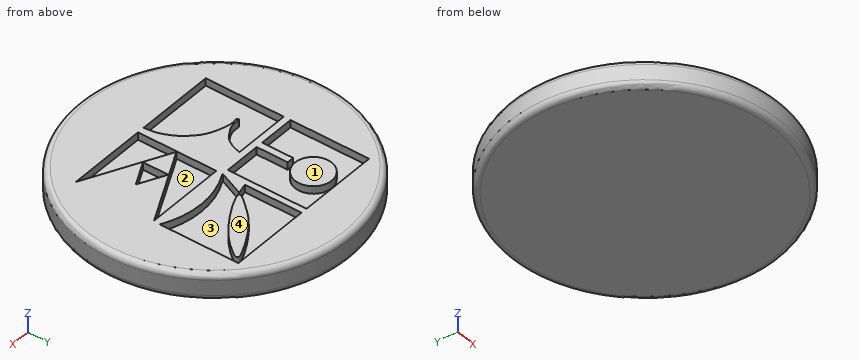
from build123d import *

# Parameters (mm, degrees)
F1_R      = 12.125
F1_W      = 7.0986367516
F1_H      = 7.0182182118
F2_DEPTH  = 2.38
F3_R      = 0.5
F4_R      = 0.5
F1_W_2    = 0.6225926336
F1_H_2    = 2.7800722164
F1_R_2    = 1.6491882735
F5_DEPTH  = 1.7
F6_DEPTH  = 2.38
F7_DEPTH  = 1.7
F8_DEPTH  = 2.38
F9_DEPTH  = 1.7
F10_DEPTH = 2.38
F11_DEPTH = 1.7
F12_DEPTH = 2.38


# Not quite as in the source:
# - a feature names something its author has since deleted; it is built from what else it names


with BuildPart() as f2:
    # F1 (on Top) → F2 (new body)
    with BuildSketch(Plane.XY):
        Circle(F1_R)
        Polygon((-7.4228290468, -6.6703339335), (-7.4228290468, 0.3279154543), (-2.3676725104, 0.3279154543), (-0.2785333199, 0.3279154543), (-0.2785333199, -6.6703339335), (-0.3460554872, -6.6703339335), align=None, mode=Mode.SUBTRACT)
        with Locations((3.8493661203, -3.1612248276)):
            Rectangle(F1_W, F1_H, mode=Mode.SUBTRACT)
        Polygon((-7.4221123941, 0.9262498352), (-7.4221123941, 7.9733738676), (-0.2785333199, 7.9733738676), (-0.2785333199, 0.9262498352), (-3.5664748866, 0.9262498352), (-4.1890675202, 0.9262498352), align=None, mode=Mode.SUBTRACT)
        Polygon((0.2827075659, 2.8855106793), (0.2827075659, 7.9663181677), (7.483521942, 7.9663181677), (7.483521942, 0.9262498352), (0.3603694204, 0.9262498352), (0.2827075659, 0.9262498352), align=None, mode=Mode.SUBTRACT)
    extrude(amount=F2_DEPTH)

    # F3
    f3_edges = [f2.edges().sort_by_distance(p)[0] for p in [
        (-12.125, 0, 2.38),
    ]]
    fillet(f3_edges, radius=F3_R)

    # F4
    f4_edges = [f2.edges().sort_by_distance(p)[0] for p in [
        (-12.125, 0, 0),
    ]]
    fillet(f4_edges, radius=F4_R)

    # F1 (on Top) → F5 (join)
    with BuildSketch(Plane.XY):
        with Locations((-3.8777712034, 2.3162859434)):
            Rectangle(F1_W_2, F1_H_2)
        Polygon((-0.2785333199, 7.9733738676), (-7.4221123941, 7.9733738676), (-7.4221123941, 0.9262498352), (-4.1890675202, 0.9262498352), (-4.1890675202, 3.7063220516), (-3.5664748866, 3.7063220516), (-3.5664748866, 0.9262498352), (-0.2785333199, 0.9262498352), align=None)
        with Locations((-3.8649578562, 5.7759984099)):
            Circle(F1_R_2, mode=Mode.SUBTRACT)
        with Locations((-3.8649578562, 5.7759984099)):
            Circle(F1_R_2)
    extrude(amount=F5_DEPTH)

    # F1 (on Top) → F6 (join, through all)
    with BuildSketch(Plane.XY):
        with Locations((-3.8649578562, 5.7759984099)):
            Circle(F1_R_2)
        with Locations((-3.8777712034, 2.3162859434)):
            Rectangle(F1_W_2, F1_H_2)
    extrude(amount=F6_DEPTH)

    # F1 (on Top) → F7 (join)
    with BuildSketch(Plane.XY):
        Polygon((7.3986844961, 0.3478842783), (0.3000477445, 0.3478842783), (0.3000477445, -6.6703339335), (7.3986844961, -6.6703339335), (0.3533055715, -3.1787578482), align=None)
        Polygon((7.3986844961, -6.6703339335), (7.3986844961, 0.3478842783), (0.3533055715, -3.1787578482), align=None)
        Polygon((2.7262428775, -4.3149543926), (2.7262428775, -2.0406346302), (5.0051301037, -3.174232257), align=None, mode=Mode.SUBTRACT)
        Polygon((5.0051301037, -3.174232257), (2.7262428775, -2.0406346302), (2.7262428775, -4.3149543926), align=None)
    extrude(amount=F7_DEPTH)

    # F1 (on Top) → F8 (join, through all)
    with BuildSketch(Plane.XY):
        Polygon((7.3986844961, -6.6703339335), (7.3986844961, 0.3478842783), (0.3533055715, -3.1787578482), align=None)
        Polygon((2.7262428775, -4.3149543926), (2.7262428775, -2.0406346302), (5.0051301037, -3.174232257), align=None, mode=Mode.SUBTRACT)
    extrude(amount=F8_DEPTH)

    # F1 (on Top) → F9 (join)
    with BuildSketch(Plane.XY):
        with BuildLine():
            Line((7.483521942, 7.9663181677), (0.2827075659, 7.9663181677))
            Line((0.2827075659, 7.9663181677), (0.2827075659, 2.8855106793))
            Line((0.2827075659, 2.8855106793), (1.2191495625, 3.121049609))
            Line((1.2191495625, 3.121049609), (0.2827075659, 0.9262498352))
            Line((0.2827075659, 0.9262498352), (0.3603694204, 0.9262498352))
            ThreePointArc((0.3603694204, 0.9262498352), (3.9219456812, 1.8291393853), (7.483521942, 0.9262498352))
            Line((7.483521942, 0.9262498352), (7.483521942, 7.9663181677))
        make_face()
        with BuildLine():
            add(Edge.make_bspline(
                [(1.3767119963, 3.2667766791), (1.2845749547, 3.4219093882), (2.4235264698, 4.7283232609), (3.5408753586, 5.9956475692), (6.2391393141, 7.418797197), (6.8917216898, 7.5995638626), (6.9665371868, 7.5324135615), (7.0858412946, 7.3423232683), (6.6731021166, 6.7922406039), (5.7276068284, 5.5974675028), (3.4869356373, 3.9709181084), (1.4800923213, 3.0927134618), (1.3767119963, 3.2667766791)],
                knots=[0, 0, 0, 0, 0.1118483914, 0.24448623, 0.4022164571, 0.4698846563, 0.4939539155, 0.5310056289, 0.6004556126, 0.7122838549, 0.8745029919, 1, 1, 1, 1], degree=3))
        make_face(mode=Mode.SUBTRACT)
        with BuildLine():
            add(Edge.make_bspline(
                [(1.3767119963, 3.2667766791), (1.2845749547, 3.4219093882), (2.4235264698, 4.7283232609), (3.5408753586, 5.9956475692), (6.2391393141, 7.418797197), (6.8917216898, 7.5995638626), (6.9665371868, 7.5324135615), (7.0858412946, 7.3423232683), (6.6731021166, 6.7922406039), (5.7276068284, 5.5974675028), (3.4869356373, 3.9709181084), (1.4800923213, 3.0927134618), (1.3767119963, 3.2667766791)],
                knots=[0, 0, 0, 0, 0.1118483914, 0.24448623, 0.4022164571, 0.4698846563, 0.4939539155, 0.5310056289, 0.6004556126, 0.7122838549, 0.8745029919, 1, 1, 1, 1], degree=3))
        make_face()
        with BuildLine():
            Line((0.3603694204, 0.9262498352), (7.483521942, 0.9262498352))
            ThreePointArc((7.483521942, 0.9262498352), (3.9219456812, 1.8291393853), (0.3603694204, 0.9262498352))
        make_face()
        Polygon((1.2191495625, 3.121049609), (0.2827075659, 2.8855106793), (0.2827075659, 0.9262498352), align=None)
    extrude(amount=F9_DEPTH)

    # F1 (on Top) → F10 (join, through all)
    with BuildSketch(Plane.XY):
        Polygon((1.2191495625, 3.121049609), (0.2827075659, 2.8855106793), (0.2827075659, 0.9262498352), align=None)
        with BuildLine():
            Line((0.3603694204, 0.9262498352), (7.483521942, 0.9262498352))
            ThreePointArc((7.483521942, 0.9262498352), (3.9219456812, 1.8291393853), (0.3603694204, 0.9262498352))
        make_face()
        with BuildLine():
            add(Edge.make_bspline(
                [(1.3767119963, 3.2667766791), (1.2845749547, 3.4219093882), (2.4235264698, 4.7283232609), (3.5408753586, 5.9956475692), (6.2391393141, 7.418797197), (6.8917216898, 7.5995638626), (6.9665371868, 7.5324135615), (7.0858412946, 7.3423232683), (6.6731021166, 6.7922406039), (5.7276068284, 5.5974675028), (3.4869356373, 3.9709181084), (1.4800923213, 3.0927134618), (1.3767119963, 3.2667766791)],
                knots=[0, 0, 0, 0, 0.1118483914, 0.24448623, 0.4022164571, 0.4698846563, 0.4939539155, 0.5310056289, 0.6004556126, 0.7122838549, 0.8745029919, 1, 1, 1, 1], degree=3))
        make_face()
    extrude(amount=F10_DEPTH)

    # F1 (on Top) → F11 (join)
    with BuildSketch(Plane.XY):
        with BuildLine():
            Line((-2.3676725104, 0.3279154543), (-7.4228290468, 0.3279154543))
            Line((-7.4228290468, 0.3279154543), (-7.4228290468, -6.6703339335))
            Line((-7.4228290468, -6.6703339335), (-0.3460554872, -6.6703339335))
            add(Edge.make_bspline(
                [(-2.3676725104, 0.3279154543), (-2.4010776229, 0.1925208975), (-2.4676626782, -0.0773555796), (-2.5876283556, -0.4592288495), (-2.8925989526, -0.9591658513), (-3.1522335022, -1.2984425332), (-3.7077309843, -1.5983279611), (-3.9910833592, -1.8042724956), (-4.6138242999, -2.0322850474), (-5.2750707973, -1.9267077545), (-5.2495717166, -2.0402242976), (-5.2345405936, -2.0988768979), (-5.1450714886, -2.160796158), (-4.6968573849, -2.0831274685), (-4.1628510391, -2.1198506981), (-2.7612179261, -2.5768069629), (-1.9266213932, -3.2203760963), (-1.1791410617, -4.0827112095), (-0.8290586767, -4.6976898082), (-0.4695580442, -5.5403229192), (-0.4210791981, -6.0329268408), (-0.3569856889, -6.488706617), (-0.3490962485, -6.6198055594), (-0.3460554872, -6.6703339335)],
                knots=[0, 0, 0, 0, 0.0435833884, 0.086873, 0.1381261489, 0.1834527151, 0.2360140714, 0.2766814959, 0.3332809415, 0.3847393962, 0.400679245, 0.417088421, 0.4369598891, 0.4804923093, 0.5317269995, 0.6128329106, 0.6846024733, 0.7554901569, 0.8138428178, 0.8776633918, 0.9266412888, 0.9717259625, 1, 1, 1, 1], degree=3))
        make_face()
        with BuildLine():
            Line((-0.2785333199, 0.3279154543), (-2.3676725104, 0.3279154543))
            add(Edge.make_bspline(
                [(-2.3676725104, 0.3279154543), (-2.4010776229, 0.1925208975), (-2.4676626782, -0.0773555796), (-2.5876283556, -0.4592288495), (-2.8925989526, -0.9591658513), (-3.1522335022, -1.2984425332), (-3.7077309843, -1.5983279611), (-3.9910833592, -1.8042724956), (-4.6138242999, -2.0322850474), (-5.2750707973, -1.9267077545), (-5.2495717166, -2.0402242976), (-5.2345405936, -2.0988768979), (-5.1450714886, -2.160796158), (-4.6968573849, -2.0831274685), (-4.1628510391, -2.1198506981), (-2.7612179261, -2.5768069629), (-1.9266213932, -3.2203760963), (-1.1791410617, -4.0827112095), (-0.8290586767, -4.6976898082), (-0.4695580442, -5.5403229192), (-0.4210791981, -6.0329268408), (-0.3569856889, -6.488706617), (-0.3490962485, -6.6198055594), (-0.3460554872, -6.6703339335)],
                knots=[0, 0, 0, 0, 0.0435833884, 0.086873, 0.1381261489, 0.1834527151, 0.2360140714, 0.2766814959, 0.3332809415, 0.3847393962, 0.400679245, 0.417088421, 0.4369598891, 0.4804923093, 0.5317269995, 0.6128329106, 0.6846024733, 0.7554901569, 0.8138428178, 0.8776633918, 0.9266412888, 0.9717259625, 1, 1, 1, 1], degree=3))
            Line((-0.3460554872, -6.6703339335), (-0.2785333199, -6.6703339335))
            Line((-0.2785333199, -6.6703339335), (-0.2785333199, 0.3279154543))
        make_face()
    extrude(amount=F11_DEPTH)

    # F1 (on Top) → F12 (join, through all)
    with BuildSketch(Plane.XY):
        with BuildLine():
            Line((-0.2785333199, 0.3279154543), (-2.3676725104, 0.3279154543))
            add(Edge.make_bspline(
                [(-2.3676725104, 0.3279154543), (-2.4010776229, 0.1925208975), (-2.4676626782, -0.0773555796), (-2.5876283556, -0.4592288495), (-2.8925989526, -0.9591658513), (-3.1522335022, -1.2984425332), (-3.7077309843, -1.5983279611), (-3.9910833592, -1.8042724956), (-4.6138242999, -2.0322850474), (-5.2750707973, -1.9267077545), (-5.2495717166, -2.0402242976), (-5.2345405936, -2.0988768979), (-5.1450714886, -2.160796158), (-4.6968573849, -2.0831274685), (-4.1628510391, -2.1198506981), (-2.7612179261, -2.5768069629), (-1.9266213932, -3.2203760963), (-1.1791410617, -4.0827112095), (-0.8290586767, -4.6976898082), (-0.4695580442, -5.5403229192), (-0.4210791981, -6.0329268408), (-0.3569856889, -6.488706617), (-0.3490962485, -6.6198055594), (-0.3460554872, -6.6703339335)],
                knots=[0, 0, 0, 0, 0.0435833884, 0.086873, 0.1381261489, 0.1834527151, 0.2360140714, 0.2766814959, 0.3332809415, 0.3847393962, 0.400679245, 0.417088421, 0.4369598891, 0.4804923093, 0.5317269995, 0.6128329106, 0.6846024733, 0.7554901569, 0.8138428178, 0.8776633918, 0.9266412888, 0.9717259625, 1, 1, 1, 1], degree=3))
            Line((-0.3460554872, -6.6703339335), (-0.2785333199, -6.6703339335))
            Line((-0.2785333199, -6.6703339335), (-0.2785333199, 0.3279154543))
        make_face()
    extrude(amount=F12_DEPTH)


solid = f2.part
Input: part model. Units: mm. Frame: model coordinates. Face numbers are marked on the shaded views. A direction names the side the tool comes from. Give positions to 0.01 mm unless a question says otherwise; leave off trailing zeros. Write each loop counter-clockwise with the first axis right and the second up, starting at its lowest first coordinate (ties: lowest second). Pieces come first, ordered by that corner, then holes. Notation, with made-up numbers: M 42,54.25 L 70,54.25 A7 ccw 70,65.25 Z; hole C 87,72 d7. An arc over 180 degrees is marked long. Use one line per item in the form item = value.
1. Cut plane A-A on z = 0.9. Return loops of the section in (x, y) (3 decimals), and give its area (3 significant figures).
Outcome:
outline = C 0,0 d24.25
area = 462 mm²
2. Mould query, pull axis X, two halves, no side actions, for the marked faces 3 and 4. Classes: released by +X, released by -X, zero draft, split by the parting line, or undercut.
Outcome:
face_3 = undercut
face_4 = zero draft
3. Reachability of the marked faces 1 and 2 from +Z, -Z, +X, -X, +Y, -Y: full face, straight path, thin tool, end or side. Return the list, or none.
Outcome:
face_1 = +Z, +X, -X, +Y, -Y
face_2 = +Z
4. Ray query, L1, parallel to X at y = -0.5, z = 2.2; L2, parallel to X at y = 5, z = 2; L3, parallel to Z at x = 2.75, y = -6. Return the intervals inside material, ascending.
Outcome:
L1 = -12 to -7.42, -2.63 to 0.3, 5.7 to 12
L2 = -11.03 to -7.42, -5.32 to -2.41, -0.28 to 0.28, 2.67 to 4.85, 7.48 to 11.03
L3 = 0 to 1.7
5. First-contact query: P1, Ø0.7, axis at y = -4, z = 2, coming from the +X side; P2, Ø0.5, axis at x = 2.5, z = 2, coming from the +Y side; P3, Ø0.7, axis at y = -3, z = 2, coming from the +X side. Flat tips, straight axial feed; report the tip coordinate or a pass-through.
Outcome:
P1 = 11.56
P2 = 11.91
P3 = 11.83
